```python
from build123d import *

# Parameters (mm, degrees)
SKETCH_W        = 90
SKETCH_H        = 115
PAD_DEPTH       = 24
SKETCH137_W     = 85.999994
SKETCH137_H     = 20
POCKET_DEPTH    = 113
FILLET_R        = 9
FILLET001_R     = 5
FILLET002_R     = 2
SKETCH143_W     = 18.3
SKETCH143_H     = 4.3
POCKET027_DEPTH = 2
FILLET004_R     = 2


with BuildPart() as part:
    # Sketch → Pad (new body)
    with BuildSketch(Plane.XY):
        with Locations((445, 157.5)):
            Rectangle(SKETCH_W, SKETCH_H)
    extrude(amount=PAD_DEPTH)

    # Sketch137 (on Face1 of Pad) → Pocket (cut)
    with BuildSketch(Plane.XZ.offset(-100)):
        with Locations((445.000003, 12)):
            Rectangle(SKETCH137_W, SKETCH137_H)
    extrude(amount=-POCKET_DEPTH, mode=Mode.SUBTRACT)

    # Fillet
    fillet_edges = [part.edges().sort_by_distance(p)[0] for p in [
        (490, 157.5, 24),
        (488, 156.5, 22),
        (402.000006, 156.5, 22),
        (400, 157.5, 24),
    ]]
    fillet(fillet_edges, radius=FILLET_R)

    # Fillet001
    fillet001_edges = [part.edges().sort_by_distance(p)[0] for p in [
        (402.000006, 156.5, 2),
        (490, 157.5, 0),
        (488, 156.5, 2),
        (400, 157.5, 0),
    ]]
    fillet(fillet001_edges, radius=FILLET001_R)

    # Fillet002
    fillet002_edges = [part.edges().sort_by_distance(p)[0] for p in [
        (445, 215, 24),
        (402.636039, 215, 21.363961),
        (400, 215, 10),
    ]]
    fillet(fillet002_edges, radius=FILLET002_R)

    # Sketch143 (on Face9 of Fillet002) → Pocket027 (cut)
    with BuildSketch(Plane(origin=(0, 215, 0), x_dir=(-1, 0, 0), z_dir=(0, 1, 0))):
        with Locations((-445, 12)):
            Rectangle(SKETCH143_W, SKETCH143_H)
    extrude(amount=-POCKET027_DEPTH, mode=Mode.SUBTRACT)

    # Fillet004
    fillet004_edges = [part.edges().sort_by_distance(p)[0] for p in [
        (435.85, 214, 9.85),
        (435.85, 214, 14.15),
        (454.15, 214, 9.85),
        (454.15, 214, 14.15),
    ]]
    fillet(fillet004_edges, radius=FILLET004_R)


with BuildPart() as part_1:
    # Body placement: moved
    add(part.part.moved(Location((0, -1, 0.25))))


solid = part_1.part
```
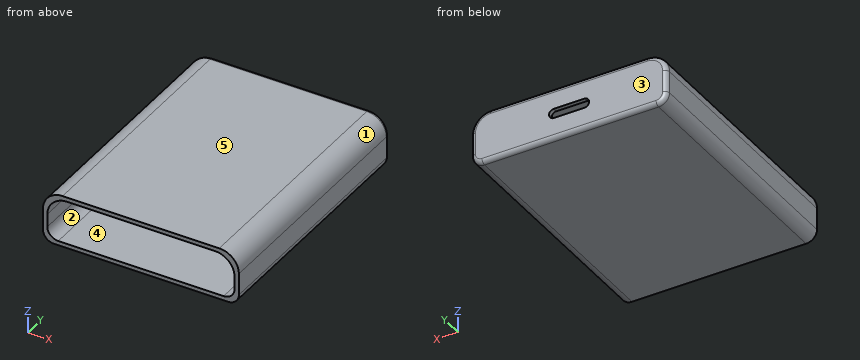
Check sheet for the modelled part. Datum: model origin and axes. Units: mm. Face numbers are marked on the shaded views. A direction names the side the tool comes from. Give positions to 0.01 mm unless a question says otherwise; leave off trailing zeros. Write each loop counter-clockwise with the first axis right and the second up, starting at its lowest first coordinate (ties: lowest second). Pieces come first, ordered by that corner, then holes.
Item 1: Gauge pin test, flat ends, axial feed: pin 1 (0.6 mm diameter, centred on x = 444.5, y = 213.5, fed in from +Z); pin 2 (2 mm diameter, centred on y = 121.5, z = 17.5, fed in from -X); pin 3 (0.6 mm diameter, centred on x = 443.5, y = 213.5, fed in from -Z); pin 4 (10 mm diameter, centred on y = 143, z = 16, fed in from +X). Record the tip position at first contact, or that the pin passes through.
Item 2: Cross-section at C-C (x = 464). Enter the section's corners in (y, z).
Item 3: Cross-section at A-A (x = 445). Enter the section's corners in (y, z).
Item 4: Access from +Z, -Z, +X, -X, +Y, -Y to the whole of each face (thin tool, end or side, straight path). Record for the marked faces 4 and 5.
Item 5: Scan lines: L1, parallel to X at y = 153.5, z = 7; L2, parallel to Z at x = 475.5, y = 190.5; L3, parallel to X at y = 209, z = 21.5. Record each from-to range of solid material in increasing order.
Item 6: Draft check along X on the marked faces 1, 2 and 3. Enter one of: released by +X, released by -X, zero draft, split by the parting line, or undercut.
Item 7: Cross-section at B-B (y = 132). Enter the section's corners in (x, z).
Report:
1. pin 1: stops at z = 23.85
1. pin 2: stops at x = 400.09
1. pin 3: stops at z = 0.65
1. pin 4: stops at x = 490
2. outline: (99, 0.25) - (212, 0.25) arc R2 ccw to (214, 2.25) - (214, 22.25) arc R2 ccw to (212, 24.25) - (99, 24.25) - (99, 22.25) - (212, 22.25) - (212, 2.25) - (99, 2.25) - close
3. outline: (99, 0.25) - (212, 0.25) arc R2 ccw to (214, 2.25) - (214, 10.1) - (212, 10.1) - (212, 2.25) - (99, 2.25) - close; (99, 22.25) - (212, 22.25) - (212, 14.4) - (214, 14.4) - (214, 22.25) arc R2 ccw to (212, 24.25) - (99, 24.25) - close
4. face 4: -Y
4. face 5: +Z, +X, -X, +Y, -Y
5. L1: x = 400 to 402.01, 487.99 to 490
5. L2: z = 0.25 to 2.25, 22.25 to 24.25
5. L3: x = 402.52 to 407.4, 482.6 to 487.48
6. face 1: released by +X
6. face 2: undercut
6. face 3: zero draft
7. outline: (400, 5.25) arc R5 ccw to (405, 0.25) - (485, 0.25) arc R5 ccw to (490, 5.25) - (490, 15.25) arc R9 ccw to (481, 24.25) - (409, 24.25) arc R9 ccw to (400, 15.25) - close; hole (402, 7.25) arc R5 ccw to (407, 2.25) - (483, 2.25) arc R5 ccw to (488, 7.25) - (488, 13.25) arc R9 ccw to (479, 22.25) - (411, 22.25) arc R9 ccw to (402, 13.25) - close
